```python
from build123d import *

# Parameters (mm, degrees)
SKETCH_1_R          = 4
SKETCH_1_R_2        = 2.5
EXTRUDE_1_DEPTH     = 10
SKETCH_2_R          = 4.3
CUT_EXTRUDE_1_DEPTH = 5


with BuildPart() as part:
    # 草图1 → 凸台-拉伸1 (new body)
    with BuildSketch(Plane.XY):
        with BuildLine():
            Line((-10, -14), (-10, -8))
            Line((-10, -8), (-17.859724479, -5.17604336))
            ThreePointArc((-17.859724479, -5.17604336), (-21.497538815, 0.16452044), (-17.546875, 5.277989933))
            Line((-17.546875, 5.277989933), (-2.8125, 9.596345333))
            ThreePointArc((-2.8125, 9.596345333), (0, 10), (2.8125, 9.596345333))
            Line((2.8125, 9.596345333), (17.546875, 5.277989933))
            ThreePointArc((17.546875, 5.277989933), (21.497538815, 0.16452044), (17.859724479, -5.17604336))
            Line((17.859724479, -5.17604336), (10, -8))
            Line((10, -8), (10, -14))
            Line((10, -14), (-10, -14))
        make_face()
        Circle(SKETCH_1_R, mode=Mode.SUBTRACT)
        with Locations((-16, 0)):
            Circle(SKETCH_1_R_2, mode=Mode.SUBTRACT)
        with Locations(Location((16, 0, 0), (0, 0, 180))):
            Circle(SKETCH_1_R_2, mode=Mode.SUBTRACT)
    extrude(amount=EXTRUDE_1_DEPTH)

    # 草图2 → 切除-拉伸1 (cut)
    with BuildSketch(Plane.XY.offset(10)):
        with Locations((-16, 0)):
            Circle(SKETCH_2_R)
        with Locations((16, 0)):
            Circle(SKETCH_2_R)
    extrude(amount=-CUT_EXTRUDE_1_DEPTH, mode=Mode.SUBTRACT)


solid = part.part
```
The listing builds one solid part. Answer for the finished solid, in the listing's coordinates (mm). A direction names the side the tool comes from. Coordinates: 2 decimals unless noted, no trailing zeros. Write each loop counter-clockwise with the first axis right and the second up, starting at its lowest first coordinate (ties: lowest second). Pieces come first, ordered by that corner, then holes. Notation, with made-up numbers: (87, 81.25) -> (121, 81.25) arc R28 ccw to (121, 111.25) -> close; hole circle Ø10 at (20, 69.5). An arc over 180 degrees is marked (long way). Write each question's results on one line, items separated by ' | '. Start each with the question number.
1) A cutting plane is placed at B-B (x = 0). Determine the outline of the cut face in (y, z).
2) Straight lines are drawn through the part: probe 1 along Y at (x, z) = (0, 7.5); probe 2 along X at (y, z) = (-8.5, 4.5); probe 3 along Y at (x, z) = (-16, 3.05). For each, find the intervals that lie inside material, in ascending order.
3) A tool of negligible diameter and unlimited length cuts with its end or side. For faces 1 (the flat face through (-14, -2, 5)), 2 (the flat face through (-10, -11, 5)), 3 (the flat face through (0, -14, 5)), from which of +Z, -Z, +X, -X, +Y, -Y can it reach the whole face along a straight path? Write none if from no direction.
4) For a pull along X with two mould halves and no side action, classify faces 4 (the cylindrical face through (-12.03, -1.65, 7.54)), 5 (the flat face through (-13.9, -6.6, 4.9)), 6 (the flat face through (10, -11, 5)) as +X half, -X half, draft (parallel to the pull), parting line (faces both ways), or undercut.
5) A cutting plane is placed at D-D (y = -6.75). Determine the outline of the cut face in (x, z).
6) A cutting plane is placed at C-C (y = 0). Determine the outline of the cut face in (x, z), then the cut area to 3 significant figures.
7) Flat-ended cylindrical pins translate along their axes: pin 1 Ø1.5 at (y, z) = (-9.5, 5.5) entering from +X; pin 2 Ø6 at (x, z) = (-10, 6.5) entering from +Y; pin 3 Ø7 at (x, y) = (0, 0) entering from +Z; pin 4 Ø8 at (x, y) = (16, 0) entering from +Z. Find the tip coordinate at first contact, or state that the pin passes through.
8) A cutting plane is placed at A-A (z = 5.5). Determine the outline of the cut face in (x, y), then the cut area to 3 significant figures.
Values follow:
1) outline: (-14, 0) -> (-4, 0) -> (-4, 10) -> (-14, 10) -> close; (4, 0) -> (10, 0) -> (10, 10) -> (4, 10) -> close
2) probe 1: -14 to -4, 4 to 10 | probe 2: -10 to 10 | probe 3: -5.84 to -2.5, 2.5 to 5.73
3) face 1: +Z | face 2: +Z, -Z, -X, -Y | face 3: +Z, -Z, +X, -X, -Y
4) face 4: undercut | face 5: -X half | face 6: +X half
5) outline: (-13.48, 0) -> (13.48, 0) -> (13.48, 10) -> (-13.48, 10) -> close
6) outline: (-21.5, 0) -> (-18.5, 0) -> (-18.5, 5) -> (-20.3, 5) -> (-20.3, 10) -> (-21.5, 10) -> close; (-13.5, 0) -> (-4, 0) -> (-4, 10) -> (-11.7, 10) -> (-11.7, 5) -> (-13.5, 5) -> close; (4, 0) -> (13.5, 0) -> (13.5, 5) -> (11.7, 5) -> (11.7, 10) -> (4, 10) -> close; (18.5, 0) -> (21.5, 0) -> (21.5, 10) -> (20.3, 10) -> (20.3, 5) -> (18.5, 5) -> close | area: 214 mm²
7) pin 1: x = 10 | pin 2: y = 8.37 | pin 3: through | pin 4: z = 5
8) outline: (-17.86, -5.18) -> (-10, -8) -> (-10, -14) -> (10, -14) -> (10, -8) -> (17.86, -5.18) arc R5.5 ccw to (17.55, 5.28) -> (2.81, 9.6) arc R10 ccw to (-2.81, 9.6) -> (-17.55, 5.28) arc R5.5 ccw to start; hole circle Ø8.6 at (-16, 0); hole circle Ø8 at (0, 0); hole circle Ø8.6 at (16, 0) | area: 550 mm²
